The listing builds one solid part. Answer for the finished solid, in the listing's coordinates (mm). Face numbers are marked on the shaded views. A direction names the side the tool comes from. Round coordinates to 2 decimals unless told otherwise and drop trailing zeros. Order: outer loops, then holes, each group sorted by start corner. A loop starts at its lowest first (then second) coordinate and runs counter-clockwise, first axis right, second up. Notation, with made-up numbers: (9.5, -16.75) - (22.5, -16.75) arc R30 ccw to (22.5, 11.25) - close; hole circle Ø5 at (45.25, -40). An arc over 180 degrees is marked (long way). One line per item, written item: value. Start each with the question number.
1. A tool of negligible diameter and unlimited length cuts with its end or side. For the marked faces 1 and 2, from which of +Z, -Z, +X, -X, +Y, -Y can it reach the whole face along a straight path? Write none if from no direction.
2. Straight lines are drawn through the part: line 1 (X direction, y = -0.1, z = 15); line 2 (Z direction, x = -1.1, y = -1); line 3 (Z direction, x = 0.15, y = 1.7). For each, find the intervals that lie inside material, in ascending order.
3. Flat-ended cylindrical pins translate along their axes: P1, Ø1, axis at x = 1, y = -1, coming from the +Z side; P2, Ø1, axis at y = 0.5, z = 17.5, coming from the +X side; P3, Ø1.3, axis at x = 1, y = -0.5, coming from the +Z side. Find the tip coordinate at first contact, or state that the pin passes through.
4. Section A-A, the plane z = 9.75 is taken. Give the vertices of the cut face in (x, y), then the cut area to 3 significant figures.
from build123d import *


with BuildPart() as part:
    # Sketch1 → Revolve1 (revolve)
    with BuildSketch(Plane(origin=(0, 0, 0), x_dir=(1, 0, 0), z_dir=(0, 1, 0))):
        with BuildLine():
            Line((0.5, -23), (2, -20.401923789))
            Line((2, -20.401923789), (2, -10.25))
            ThreePointArc((2, -10.25), (2.014644661, -10.214644661), (2.05, -10.2))
            Line((2.05, -10.2), (2.2, -10.2))
            Line((2.2, -10.2), (2.2, -9.349807217))
            Line((2.2, -9.349807217), (1.309042398, -8.077387893))
            ThreePointArc((1.309042398, -8.077387893), (1.305649458, -8.025621641), (1.35, -7.998709071))
            Line((1.35, -7.998709071), (2.2, -7.998709071))
            Line((2.2, -7.998709071), (2.2, -7.748709071))
            Line((2.2, -7.748709071), (2.009042398, -7.475993352))
            ThreePointArc((2.009042398, -7.475993352), (2.002314152, -7.462349821), (2, -7.447314531))
            Line((2, -7.447314531), (2, 0))
            Line((2, 0), (1, 0))
            Line((1, 0), (1, -21.49956969))
            Line((1, -21.49956969), (0.5, -21.8))
            Line((0.5, -21.8), (0.5, -22.419741814))
            Line((0.5, -22.419741814), (0.2, -22.6))
            Line((0.2, -22.6), (0.2, -23))
            Line((0.2, -23), (0.5, -23))
        make_face()
    revolve(axis=Axis((0, 0, 0), (0, 0, 1)))


solid = part.part
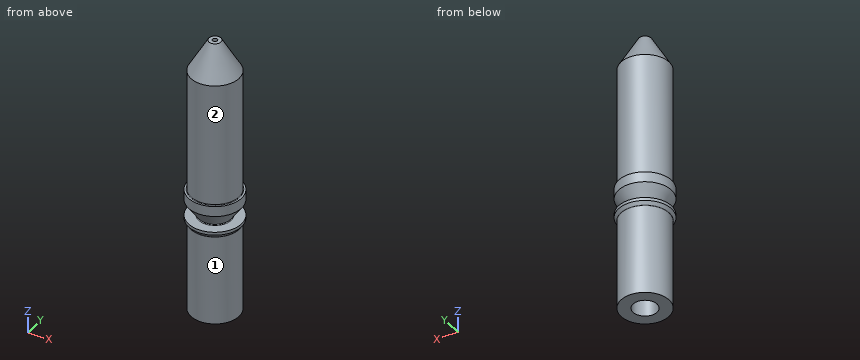
Answer list:
1. face 1: -Z
1. face 2: +Z
2. line 1: x = -2 to -0.99, 0.99 to 2
2. line 2: z = 0 to 8, 8.33 to 21.29
2. line 3: z = 0 to 8, 8.65 to 20.91
3. P1: stops at z = 22.28
3. P2: stops at x = 2
3. P3: stops at z = 23
4. outline: circle Ø4.4 at (0, 0); hole circle Ø2 at (0, 0)
4. area: 12.1 mm²
